Read the model definition and answer for the solid it produces. Units are mm, in the model's axes. Coordinates: 2 decimals unless noted, no trailing zeros. Loops run counter-clockwise (first coordinate to the right, second up) from the corner with the lowest first, then second, coordinate; pieces in that order, holes last. Notation, with made-up numbers: M -38,53 L -32,53 A17 ccw -32,76 Z; hole C 66,55.25 d7. An arc over 180 degrees is marked long. Put each result on its own line as item: value.
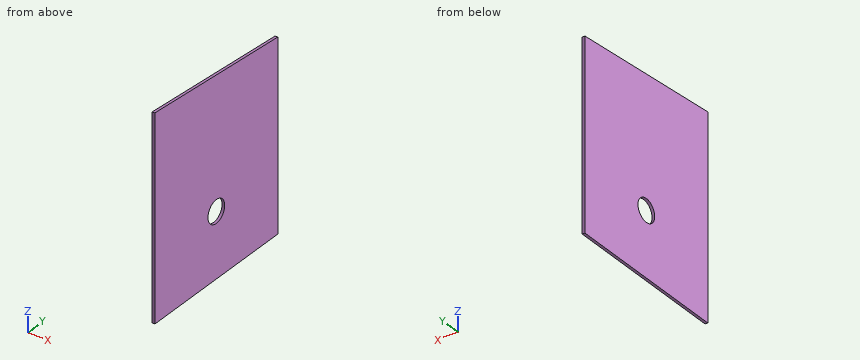
from build123d import *

# Parameters (mm, degrees)
F0_R     = 17
F1_DEPTH = 4


with BuildPart() as f1:
    # F0 (on Right) → F1 (new body)
    with BuildSketch(Plane.YZ):
        Polygon((-125, 300), (-125, 0), (125, 0), (125, 280), align=None)
        with Locations((0, 96)):
            Circle(F0_R, mode=Mode.SUBTRACT)
    extrude(amount=F1_DEPTH)


solid = f1.part
1) Find section B-B, the plane x = 2.8. Write down the section's boundary in (y, z), plus the area to 3 significant figures.
Answer list:
outline: M -125,0 L 125,0 L 125,280 L -125,300 Z; hole C 0,96 d34
area: 71,600 mm^2
2) Find section C-C, the plane z = 96. Write down the section's boundary in (x, y).
Answer list:
outline: M 0,-125 L 4,-125 L 4,-17 L 0,-17 Z; M 0,17 L 4,17 L 4,125 L 0,125 Z
3) Given pin 1 Ø1 at (x, y) = (1, 54) entering from +Z, flat-ended and moving along its own axis, determine where the tip first touches the part or whether it passes through.
Answer list:
pin 1: stops at z = 285.72
4) Straight lines are drawn through the part: line 1 (Y direction, x = 3.75, z = 95.5); line 2 (Z direction, x = 2.15, y = 0); line 3 (Z direction, x = 0.35, y = 12). For each, find the intervals that lie inside material, in ascending order. Write a range as [from, to].
Answer list:
line 1: y = [-125, -16.99], [16.99, 125]
line 2: z = [0, 79], [113, 290]
line 3: z = [0, 83.96], [108.04, 289.04]
5) Find section A-A, the plane y = 0. Write down the section's boundary in (x, z), plus the area to 3 significant figures.
Answer list:
outline: M 0,0 L 4,0 L 4,79 L 0,79 Z; M 0,113 L 4,113 L 4,290 L 0,290 Z
area: 1,020 mm^2
6) Find section D-D, the plane y = 103. Write down the section's boundary in (x, z).
Answer list:
outline: M 0,0 L 4,0 L 4,281.76 L 0,281.76 Z
